Design review of the part built by this model. Coordinates are the model's own, in mm. Face numbers are marked on the shaded views. A direction names the side the tool comes from. Round coordinates to 2 decimals unless told otherwise and drop trailing zeros. Loops run counter-clockwise (first coordinate to the right, second up) from the corner with the lowest first, then second, coordinate; pieces in that order, holes last. Notation, with made-up numbers: M 19.5,79 L 35.5,79 A29 ccw 35.5,109 Z; hole C 6.25,57.25 d10. An arc over 180 degrees is marked long. One line per item, written item: value. Start each with the question number.
Item 1: We need section D-D (y = 14). Write out the cut boundary in (x, z).
Item 2: For line 1 along X through (y, z) = (5, 3.5); line 2 along X through (y, z) = (20.5, 3.5); line 3 along X through (y, z) = (2.5, 8), list the stretches that pass through material, from the lowest coordinate up.
Item 3: We need section A-A (y = 25). Write out the cut boundary in (x, z).
Item 4: We need section C-C (x = 21.5). Write out the cut boundary in (y, z).
Item 5: For the marked faces 5, 6, 7 and 8, list the 3-axis set-ups (+Z, -Z, +X, -X, +Y, -Y) from which the entire face can be reached by the end or side of a thin tool; tool diameter is ignored.
Item 6: Clearance check with flat-ended pins moving along their axes: pin 1 (1.2 mm diameter, centred on x = 3.5, z = 4, fed in from -Y); pin 2 (6 mm diameter, centred on x = 8.5, y = 22, fed in from +Z); pin 3 (3 mm diameter, centred on x = 15, z = 1.5, fed in from -Y). State where each tip first meets the part, or that it passes through.
Item 7: We need section B-B (z = 9.5). Write out the cut boundary in (x, y), then the cut area to 4 significant figures.
Item 8: Mouldability with a two-part tool opening along Z and no side actions: class the marked faces 1, 2, 3 and 4 as released by +Z, released by -Z, zero draft, split by the parting line, or undercut.
from build123d import *

# Parameters (mm, degrees)
SKETCH_1_W          = 25
SKETCH_1_H          = 27
EXTRUDE_1_DEPTH     = 10
SKETCH_2_W          = 20.5
SKETCH_2_H          = 27
CUT_EXTRUDE_1_DEPTH = 3
SKETCH_3_R          = 1.25
CUT_EXTRUDE_2_DEPTH = 12
SKETCH_4_R          = 1.25
CUT_EXTRUDE_3_DEPTH = 12
SKETCH_5_W          = 10
SKETCH_5_H          = 10
CUT_EXTRUDE_4_DEPTH = 12
FILLET_1_R          = 3


with BuildPart() as part:
    # 스케치1 → 보스-돌출1 (new body)
    with BuildSketch(Plane.XY):
        with Locations((12.5, 13.5)):
            Rectangle(SKETCH_1_W, SKETCH_1_H)
    extrude(amount=EXTRUDE_1_DEPTH)

    # 스케치2 → 컷-돌출1 (cut)
    with BuildSketch(Plane.XY.offset(10)):
        with Locations((12.5, 13.5)):
            Rectangle(SKETCH_2_W, SKETCH_2_H)
    extrude(amount=-CUT_EXTRUDE_1_DEPTH, mode=Mode.SUBTRACT)

    # 스케치3 → 컷-돌출2 (cut)
    with BuildSketch(Plane(origin=(0, 27, 0), x_dir=(1, 0, 0), z_dir=(0, 1, 0))):
        with Locations(Location((7.5, -3.5, 0), (0, 0, 270))):
            Circle(SKETCH_3_R)
        with Locations(Location((17.5, -3.5, 0), (0, 0, 270))):
            Circle(SKETCH_3_R)
    extrude(amount=-CUT_EXTRUDE_2_DEPTH, mode=Mode.SUBTRACT)

    # 스케치4 → 컷-돌출3 (cut)
    with BuildSketch(Plane.XZ):
        with Locations(Location((3.5, 3.5, 0), (0, 0, 270))):
            Circle(SKETCH_4_R)
        with Locations(Location((21.5, 3.5, 0), (0, 0, 270))):
            Circle(SKETCH_4_R)
    extrude(amount=-CUT_EXTRUDE_3_DEPTH, mode=Mode.SUBTRACT)

    # 스케치5 → 컷-돌출4 (cut)
    with BuildSketch(Plane(origin=(0, 0, 0), x_dir=(-1, 0, 0), z_dir=(0, 0, -1))):
        with Locations((-12.5, 5)):
            Rectangle(SKETCH_5_W, SKETCH_5_H)
    extrude(amount=-CUT_EXTRUDE_4_DEPTH, mode=Mode.SUBTRACT)

    # 필렛1
    fillet_1_edges = [part.edges().sort_by_distance(p)[0] for p in [
        (25, 13.5, 0),
        (17.5, 10, 3.5),
        (7.5, 10, 3.5),
        (0, 13.5, 0),
    ]]
    fillet(fillet_1_edges, radius=FILLET_1_R)


solid = part.part
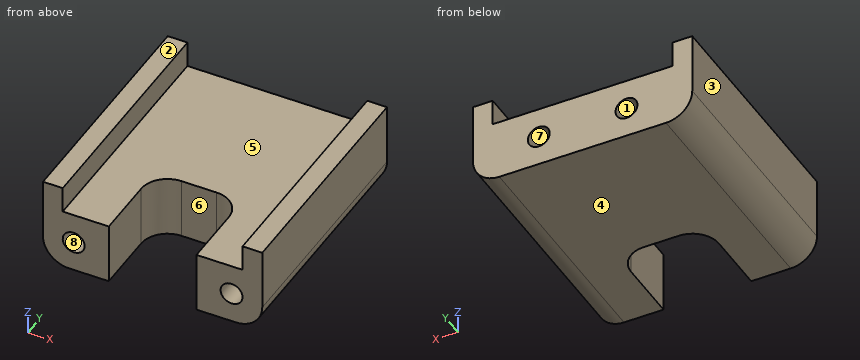
A:
1. outline: M 0,3 A3 ccw 3,0 L 22,0 A3 ccw 25,3 L 25,10 L 22.75,10 L 22.75,7 L 2.25,7 L 2.25,10 L 0,10 Z
2. line 1: 0 to 2.25, 4.75 to 7.5, 17.5 to 20.25, 22.75 to 25
2. line 2: 0 to 6.25, 8.75 to 16.25, 18.75 to 25
2. line 3: 0 to 2.25, 22.75 to 25
3. outline: M 0,3 A3 ccw 3,0 L 22,0 A3 ccw 25,3 L 25,10 L 22.75,10 L 22.75,7 L 2.25,7 L 2.25,10 L 0,10 Z; hole C 7.5,3.5 d2.5; hole C 17.5,3.5 d2.5
4. outline: M 0,0 L 27,0 L 27,7 L 0,7 L 0,4.75 L 12,4.75 L 12,2.25 L 0,2.25 Z
5. face 5: +Z, +Y, -Y
5. face 6: +Z, -Z, -Y
5. face 7: +Y
5. face 8: -Y
6. pin 1: y = 12
6. pin 2: z = 7
6. pin 3: y = 9.24
7. outline: M 0,0 L 2.25,0 L 2.25,27 L 0,27 Z; M 22.75,0 L 25,0 L 25,27 L 22.75,27 Z
7. area: 121.5 mm2
8. face 1: undercut
8. face 2: released by +Z
8. face 3: zero draft
8. face 4: released by -Z
